Model file for the job. Use its own axes, mm. A direction names the side the tool comes from. Coordinates: 2 decimals unless noted, no trailing zeros. Order: outer loops, then holes, each group sorted by start corner. A loop starts at its lowest first (then second) coordinate and runs counter-clockwise, first axis right, second up. Notation, with made-up numbers: (25.5, -25.75) -> (47.5, -25.75) arc R24 cw to (47.5, -15.75) -> close; hole circle Ø8 at (76, -22.5). An arc over 180 degrees is marked (long way). Return JSON: item names as keys, results as strings. Group by question number.
1) Cut at C-C (z = 45.5). Write the cut outline in (x, y), and give its area (3 significant figures).
2) Cut at D-D (x = -27). Write the cut outline in (y, z), and give its area (3 significant figures).
3) Cut at A-A (x = 0). State how many separate pieces and enclosed holes the cut face has, and give its area (3 significant figures).
4) Flat gauge pins, fed straight in: pin 1 (5 mm diameter, centred on y = 42.5, z = 31.5, fed in from -X); pin 2 (2.5 mm diameter, centred on x = 16, y = 155.5, fed in from -Z); pin 3 (1.7 mm diameter, centred on x = -17, y = 37, fed in from +Z); pin 4 (12 mm diameter, centred on x = 8, y = -44, fed in from +Z). Where does each tip first touch, or does it go through?
5) Pull direction Z, two halves, no side cores. Call faces 1 (the flat face through (-12, 32, 80)), 2 (the flat face through (20, -80, 15)), 3 (the flat face through (-16.056, 48.094, -9.319)), 4 (the cylindrical face through (0.176, 173.856, -25.756)): +Z half, -Z half, draft (parallel to the pull), parting line (faces both ways), or undercut.
6) Probe line 1 (Y direction, x = 0.5, z = 10); line 2 (Y direction, x = 0, z = 23); line 3 (X direction, y = 175.5, z = -21.76). List the from-to ranges inside material, lowest first.
7) Which spindle directions (+Z, -Z, +X, -X, +Y, -Y) get a long thin tool onto all of the face, cutting with end or side? Do faces 5 (the flat face through (20, 107, -2)), 6 (the flat face through (-20, 105, -2)), 7 (the flat face through (-12, 118, -10)), 8 (the flat face through (16, 78, -18.38)). Say none if no direction does.
8) Cut at B-B (y = 0). Write the cut outline in (x, z).
from build123d import *

# Parameters (mm, degrees)
SKETCH1_R            = 39
SKETCH1_R_2          = 34
BOSS_EXTRUDE1_DEPTH  = 80
BOSS_EXTRUDE2_DEPTH  = 20
BOSS_EXTRUDE3_DEPTH  = 20
BOSS_EXTRUDE4_DEPTH  = 8
BOSS_EXTRUDE5_DEPTH  = 8
CUT_EXTRUDE1_DEPTH   = 73
SKETCH13_R           = 4
CUT_EXTRUDE2_DEPTH   = 24
SKETCH14_R           = 4
CUT_EXTRUDE3_DEPTH   = 24
BOSS_EXTRUDE6_DEPTH  = 8
BOSS_EXTRUDE7_DEPTH  = 8
BOSS_EXTRUDE8_DEPTH  = 8
BOSS_EXTRUDE14_DEPTH = 8
BOSS_EXTRUDE15_DEPTH = 8
BOSS_EXTRUDE16_DEPTH = 8
BOSS_EXTRUDE17_DEPTH = 8
BOSS_EXTRUDE18_DEPTH = 26
BOSS_EXTRUDE19_REACH = 195.204


with BuildPart() as part:
    # Sketch1 → Boss-Extrude1 (new body)
    with BuildSketch(Plane.XY):
        Circle(SKETCH1_R)
        Circle(SKETCH1_R_2, mode=Mode.SUBTRACT)
    extrude(amount=BOSS_EXTRUDE1_DEPTH)



with BuildPart() as body_2:
    # Sketch3 → Boss-Extrude2 (new, symmetric)
    with BuildSketch(Plane(origin=(0, 0, 0), x_dir=(0, 0, -1), z_dir=(1, 0, 0))):
        Polygon((-8, 39), (-8, 177.8), (36.76, 177.8), (36.76, 169.8), (0, 169.8), (0, 39), align=None)
    extrude(amount=BOSS_EXTRUDE2_DEPTH, both=True)


with BuildPart() as body_3:
    # Sketch4 → Boss-Extrude3 (new, symmetric)
    with BuildSketch(Plane(origin=(0, 0, 0), x_dir=(0, 0, -1), z_dir=(1, 0, 0))):
        Polygon((-27.91, -39), (-27.91, -127), (10.09, -127), (10.09, -119), (-19.91, -119), (-19.91, -39), align=None)
    extrude(amount=BOSS_EXTRUDE3_DEPTH, both=True)


with BuildPart() as part_1:
    add(part.part)

    add(body_3.part)  # Boss-Extrude4 merges body 3
    # Sketch6 → Boss-Extrude4 (add)
    with BuildSketch(Plane(origin=(0, 0, 19.91), x_dir=(-1, 0, 0), z_dir=(0, 0, -1))):
        with BuildLine():
            ThreePointArc((20, -33.481338086), (10.373712322, -37.595027499), (0, -39))
            Line((0, -39), (20, -39))
            Line((20, -39), (20, -33.481338086))
        make_face()
        with BuildLine():
            Line((-20, -33.481338086), (-20, -39))
            Line((-20, -39), (0, -39))
            ThreePointArc((0, -39), (-10.373712322, -37.595027499), (-20, -33.481338086))
        make_face()
    extrude(amount=-BOSS_EXTRUDE4_DEPTH)


    add(body_2.part)  # Boss-Extrude5 merges body 2
    # Sketch7 → Boss-Extrude5 (add)
    with BuildSketch(Plane(origin=(0, 0, 0), x_dir=(-1, 0, 0), z_dir=(0, 0, -1))):
        with BuildLine():
            Line((0, 39), (-20, 39))
            Line((-20, 39), (-20, 33.481338086))
            ThreePointArc((-20, 33.481338086), (-10.373712322, 37.595027499), (0, 39))
        make_face()
        with BuildLine():
            Line((20, 39), (0, 39))
            ThreePointArc((0, 39), (10.373712322, 37.595027499), (20, 33.481338086))
            Line((20, 33.481338086), (20, 39))
        make_face()
    extrude(amount=-BOSS_EXTRUDE5_DEPTH)

    # Sketch12 → Cut-Extrude1 (cut)
    with BuildSketch(Plane(origin=(0, 0, 0), x_dir=(-1, 0, 0), z_dir=(0, 0, -1))):
        with BuildLine():
            Line((5.059933618, 132.933679622), (5.059933618, 86.710392146))
            ThreePointArc((5.059933618, 86.710392146), (0, 81.650458528), (-5.059933618, 86.710392146))
            Line((-5.059933618, 86.710392146), (-5.059933618, 132.933679622))
            ThreePointArc((-5.059933618, 132.933679622), (0, 137.993613239), (5.059933618, 132.933679622))
        make_face()
        with BuildLine():
            Line((4.756389645, -68.737317272), (4.756389645, -97.444530968))
            ThreePointArc((4.756389645, -97.444530968), (0, -102.200920613), (-4.756389645, -97.444530968))
            Line((-4.756389645, -97.444530968), (-4.756389645, -68.737317272))
            ThreePointArc((-4.756389645, -68.737317272), (0, -63.980927627), (4.756389645, -68.737317272))
        make_face()
    extrude(amount=-CUT_EXTRUDE1_DEPTH, mode=Mode.SUBTRACT)

    # Sketch13 → Cut-Extrude2 (cut)
    with BuildSketch(Plane(origin=(0, 177.8, 0), x_dir=(1, 0, 0), z_dir=(0, 1, 0))):
        with Locations(Location((0, 21.76, 0), (0, 0, 270))):
            Circle(SKETCH13_R)
    extrude(amount=-CUT_EXTRUDE2_DEPTH, mode=Mode.SUBTRACT)

    # Sketch14 → Cut-Extrude3 (cut)
    with BuildSketch(Plane.XZ.offset(127)):
        with Locations(Location((0, 4.91, 0), (0, 0, 270))):
            Circle(SKETCH14_R)
    extrude(amount=-CUT_EXTRUDE3_DEPTH, mode=Mode.SUBTRACT)

    # Sketch15 → Boss-Extrude6 (add)
    with BuildSketch(Plane(origin=(20, 0, 0), x_dir=(0, 0, -1), z_dir=(1, 0, 0))):
        Polygon((0, -119), (0, -99.086888853), (-4.91, -71.464610667), (-4.91, -49.814716953), (-1.4130197, -33.634678949), (-19.91, -33.481338086), (-19.91, -119), align=None)
    extrude(amount=-BOSS_EXTRUDE6_DEPTH)

    # Sketch16 → Boss-Extrude7 (add)
    with BuildSketch(Plane.ZY.offset(20)):
        Polygon((0, -119), (0, -99.086888853), (4.91, -71.464610667), (4.91, -49.814716953), (1.379878246, -33.481338086), (19.91, -33.481338086), (19.91, -119), align=None)
    extrude(amount=-BOSS_EXTRUDE7_DEPTH)

    # Sketch17 → Boss-Extrude8 (add)
    with BuildSketch(Plane(origin=(20, 0, 0), x_dir=(0, 0, -1), z_dir=(1, 0, 0))):
        Polygon((25.76, 169.8), (25.76, 143.643001818), (18.38, 94.201688411), (18.38, 62.304066859), (0, 33.481338086), (0, 169.8), align=None)
    extrude(amount=-BOSS_EXTRUDE8_DEPTH)

    # Sketch23 → Boss-Extrude14 (add)
    with BuildSketch(Plane(origin=(20, 0, 0), x_dir=(0, 0, -1), z_dir=(1, 0, 0))):
        Polygon((-8, 121.891336637), (-33.564768945, 39), (-8, 39), align=None)
        Polygon((-40, -39), (-27.91, -80.240669043), (-27.91, -39), align=None)
    extrude(amount=-BOSS_EXTRUDE14_DEPTH)

    # Sketch24 → Boss-Extrude15 (add)
    with BuildSketch(Plane.ZY.offset(20)):
        Polygon((0, 169.8), (-25.76, 169.8), (-25.76, 143.643001818), (-18.38, 94.201688411), (-18.38, 62.304066859), (0, 33.481338086), align=None)
    extrude(amount=-BOSS_EXTRUDE15_DEPTH)

    # Sketch25 → Boss-Extrude16 (add)
    with BuildSketch(Plane.ZY.offset(20)):
        Polygon((8, 39), (33.564768945, 39), (8, 121.891336637), align=None)
    extrude(amount=-BOSS_EXTRUDE16_DEPTH)

    # Sketch26 → Boss-Extrude17 (add)
    with BuildSketch(Plane.ZY.offset(20)):
        Polygon((27.91, -39), (27.91, -80.240669043), (40, -39), align=None)
    extrude(amount=-BOSS_EXTRUDE17_DEPTH)

    # Sketch28 → Boss-Extrude18 (add)
    with BuildSketch(Plane.XY.offset(8)):
        with BuildLine():
            ThreePointArc((-12, 37.107950631), (-16.102424651, 35.52058446), (-20, 33.481338086))
            Line((-20, 33.481338086), (-20, 39))
            Line((-20, 39), (-12, 39))
            Line((-12, 39), (-12, 37.107950631))
        make_face()
        with BuildLine():
            ThreePointArc((20, 33.481338086), (16.102424651, 35.52058446), (12, 37.107950631))
            Line((12, 37.107950631), (12, 39))
            Line((12, 39), (20, 39))
            Line((20, 39), (20, 33.481338086))
        make_face()
    extrude(amount=BOSS_EXTRUDE18_DEPTH)

    # Boss-Extrude19: up to this plane
    boss_extrude19_end = Plane(origin=(-12, -80.240669043, 27.91), z_dir=(0, -0.2813179552300577, 0.9596146143453523))
    # Sketch29 → Boss-Extrude19 (add, up to the surface)
    with BuildSketch(Plane.XY.offset(28), mode=Mode.PRIVATE) as boss_extrude19_sk1:
        with BuildLine():
            Line((-12, -39), (-12, -37.107950631))
            ThreePointArc((-12, -37.107950631), (-16.102424651, -35.52058446), (-20, -33.481338086))
            Line((-20, -33.481338086), (-20, -39))
            Line((-20, -39), (-12, -39))
        make_face()
    boss_extrude19_tool1 = split(extrude(boss_extrude19_sk1.sketch, amount=BOSS_EXTRUDE19_REACH, mode=Mode.PRIVATE), bisect_by=boss_extrude19_end, keep=Keep.BOTH, mode=Mode.PRIVATE)
    add(boss_extrude19_tool1.solids().sort_by_distance((-16.684032, -37.08267, 28))[0])
    # Sketch29 → Boss-Extrude19 (add, up to the surface)
    with BuildSketch(Plane.XY.offset(28), mode=Mode.PRIVATE) as boss_extrude19_sk2:
        with BuildLine():
            Line((12, -39), (12, -37.107950631))
            ThreePointArc((12, -37.107950631), (16.102424651, -35.52058446), (20, -33.481338086))
            Line((20, -33.481338086), (20, -39))
            Line((20, -39), (12, -39))
        make_face()
    boss_extrude19_tool2 = split(extrude(boss_extrude19_sk2.sketch, amount=BOSS_EXTRUDE19_REACH, mode=Mode.PRIVATE), bisect_by=boss_extrude19_end, keep=Keep.BOTH, mode=Mode.PRIVATE)
    add(boss_extrude19_tool2.solids().sort_by_distance((16.684032, -37.08267, 28))[0])


solid = part_1.part
Answers below:
{
 "1": {"outline": "circle Ø78 at (0, 0); hole circle Ø68 at (0, 0)", "area": "1,150 mm^2"},
 "2": {"outline": "(-28.14, 0) -> (-20.66, 0) -> (-20.66, 80) -> (-28.14, 80) -> close; (20.66, 0) -> (28.14, 0) -> (28.14, 80) -> (20.66, 80) -> close", "area": "1,200 mm^2"},
 "3": {"separate pieces": "6", "enclosed holes": "0", "area": "2,260 mm^2"},
 "4": {"pin 1": "stops at x = -20", "pin 2": "stops at z = -25.76", "pin 3": "stops at z = 34", "pin 4": "stops at z = 80"},
 "5": {"face 1": "+Z half", "face 2": "draft", "face 3": "-Z half", "face 4": "undercut"},
 "6": {"line 1": "y = -127 to -119, -39 to -34, 34 to 39", "line 2": "y = -127 to -102.2, -63.98 to -34, 34 to 39", "line 3": "x = -20 to -4, 4 to 20"},
 "7": {"face 5": "+Z, -Z, +X, +Y", "face 6": "+Z, -Z, -X, +Y", "face 7": "-Z", "face 8": "-Z, +X, -X, -Y"},
 "8": {"outline": "(-39, 0) -> (-34, 0) -> (-34, 80) -> (-39, 80) -> close; (34, 0) -> (39, 0) -> (39, 80) -> (34, 80) -> close"}
}
